Autodesk Inventor part; units mm, degrees
ref_plane "YZ Plane" through (0, 0, 0) normal (1, 0, 0) x (0, 1, 0)
ref_plane "XZ Plane" through (0, 0, 0) normal (0, 1, 0) x (-1, 0, 0)
ref_plane "XY Plane" through (0, 0, 0) normal (0, 0, 1) x (1, 0, 0)
sketch "Sketch1" plane through (0, 0, 0) normal (0, 0, 1) x (1, 0, 0)
  line L0 (0, 0) -> (304.8, 0)
  line L1 (304.8, 0) -> (304.8, 304.8)
  line L2 (304.8, 304.8) -> (0, 304.8)
  line L3 (0, 304.8) -> (0, 0)
  line L4 (25.4, 25.4) -> (279.4, 25.4)
  line L5 (279.4, 25.4) -> (279.4, 279.4)
  line L6 (279.4, 279.4) -> (25.4, 279.4)
  line L7 (25.4, 279.4) -> (25.4, 25.4)
  circle A0 centre (15.875, 231.15) radius 3.175
  circle A1 centre (288.673, 231.15) radius 3.175
  circle A2 centre (15.875, 73.65) radius 3.175
  circle A3 centre (288.673, 73.65) radius 3.175
  dimension "d0" = 304.8
  dimension "d1" = 304.8
  dimension "d2" = 254
  dimension "d3" = 254
  dimension "d4" = 25.4
  dimension "d5" = 25.4
  dimension "d8" = 6.35
  dimension "d9" = 73.65
  dimension "d10" = 15.875
  dimension "d13" = 272.798
  dimension "d16" = 157.5
extrude "Extrusion1" add sketch "Sketch1" along normal blind 3.175
properties part number "TurretBasePlate"
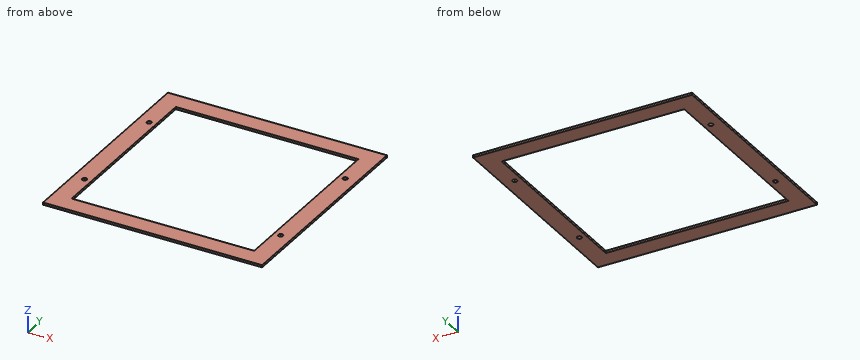
Input: part model. Units: mm. Frame: model coordinates. Coordinates: 2 decimals unless noted, no trailing zeros. Loops run counter-clockwise (first coordinate to the right, second up) from the corner with the lowest first, then second, coordinate; pieces in that order, holes last. Notation, with made-up numbers: M -36.5,47.25 L -18.5,47.25 A28 ccw -18.5,68.25 Z; hole C 45.25,-13 d7. An arc over 180 degrees is marked long. Answer in a Markdown table with one row per item.
1. Section A-A, the plane z = 1.5. Output: boundary loops of the cut face in (x, y) (3 decimals).
Response:
| item | result |
|---|---|
| outline | M 0,0 L 304.8,0 L 304.8,304.8 L 0,304.8 Z; hole C 15.875,73.65 d6.35; hole C 15.875,231.15 d6.35; hole M 25.4,25.4 L 279.4,25.4 L 279.4,279.4 L 25.4,279.4 Z; hole C 288.673,73.65 d6.35; hole C 288.673,231.15 d6.35 |
2. Material intervals for line 1 (X direction, y = 231.15, z = 2.3); line 2 (X direction, y = 262.5, z = 2.65), sorted ascending.
Response:
| item | result |
|---|---|
| line 1 | x = 0 to 12.7, 19.05 to 25.4, 279.4 to 285.5, 291.85 to 304.8 |
| line 2 | x = 0 to 25.4, 279.4 to 304.8 |
3. Section B-B, the plane y = 164. Output: boundary loops of the cut face in (x, z) (3 decimals), then the cut area to 3 significant figures.
Response:
| item | result |
|---|---|
| outline | M 0,0 L 25.4,0 L 25.4,3.175 L 0,3.175 Z; M 279.4,0 L 304.8,0 L 304.8,3.175 L 279.4,3.175 Z |
| area | 161 mm2 |
4. First-contact query: pin 1 (5 mm diameter, centred on x = 15.875, y = 231.15, fed in from +Z). Flat tip, straight axial feed; report the tip coordinate or a pass-through.
Response:
| item | result |
|---|---|
| pin 1 | passes through |
